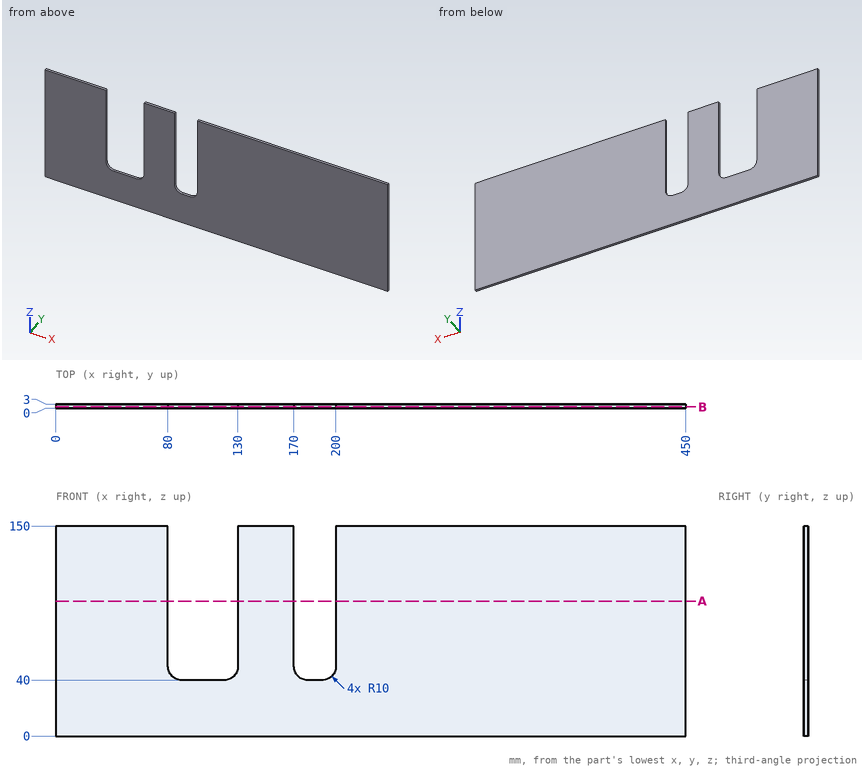
The drawing under review shows one solid part. Ordinate dimensions are in mm from its lowest x, y, z. Give positions to 0.01 mm unless a question says otherwise; leave off trailing zeros. Loops run counter-clockwise (first coordinate to the right, second up) from the corner with the lowest first, then second, coordinate; pieces in that order, holes last. Notation, with made-up numbers: M -7,-37.75 L 12,-37.75 A17 cw 12,-12.75 Z; hole C -32,-17.5 d2. An arc over 180 degrees is marked long. One line per item, written item: value. Start each with the question number.
Q1. Add section A-A (z = 96.5). Give the boundary of the cut face in (x, y), and give its area (3 significant figures).
Q2. Add section B-B (y = 1). Give the boundary of the cut face in (x, z).
Q3. Clearance check with a flat-ended pin moving along its axis: pin 1 Ø1.5 at (x, y) = (183.5, 1.5) entering from +Z. State where the tip first meets the part, or that it passes through.
Q4. For L1, parallel to X at y = 0.35, z = 85; L2, parallel to X at y = 2.05, z = 44; L3, parallel to Z at x = 122.5, y = 0.4, list the stretches that pass through material, from the lowest coordinate up.
Reply:
1. outline: M 0,0 L 80,0 L 80,3 L 0,3 Z; M 130,0 L 170,0 L 170,3 L 130,3 Z; M 200,0 L 450,0 L 450,3 L 200,3 Z
1. area: 1,110 mm²
2. outline: M 0,0 L 450,0 L 450,150 L 200,150 L 200,50 A10 cw 190,40 L 180,40 A10 cw 170,50 L 170,150 L 130,150 L 130,50 A10 cw 120,40 L 90,40 A10 cw 80,50 L 80,150 L 0,150 Z
3. pin 1: z = 40
4. L1: 0 to 80, 130 to 170, 200 to 450
4. L2: 0 to 82, 128 to 172, 198 to 450
4. L3: 0 to 40.32
